from build123d import *

# Parameters (mm, degrees)
F0_W      = 40.221851
F0_H      = 25.612304
F1_DEPTH  = 25.4
F1_FACE_W = 40.22185
F1_FACE_H = 25.612304
F2_DEPTH  = 25.4
F3_R      = 3.681994
F4_DEPTH  = 25.4


with BuildPart() as f1:
    # F0 (on Top) → F1 (new body)
    with BuildSketch(Plane.XY):
        with Locations((4.765831, -2.674487)):
            Rectangle(F0_W, F0_H)
    extrude(amount=F1_DEPTH)

    # F1_face (on face) → F2 (join)
    with BuildSketch(Plane(origin=(4.765831, -2.674487, 25.4), x_dir=(1, 0, 0), z_dir=(0, 0, 1))):
        Rectangle(F1_FACE_W, F1_FACE_H)
    extrude(amount=F2_DEPTH)

    # F3 (on face) → F4 (join)
    with BuildSketch(Plane.XZ.offset(15.480639)):
        with Locations((4.6224, 33.59535)):
            Circle(F3_R)
    extrude(amount=F4_DEPTH)


solid = f1.part
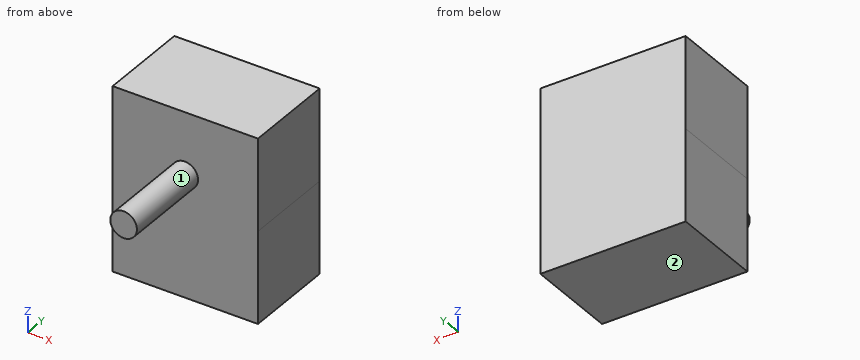
Verification items for the finished model (mm, model axes). Face numbers are marked on the shaded views. A direction names the side the tool comes from. Give positions to 0.01 mm unless a question says otherwise; leave off trailing zeros. Order: outer loops, then holes, each group sorted by start corner. A loop starts at its lowest first (then second) coordinate and runs counter-clockwise, first axis right, second up. Notation, with made-up numbers: M 82,20 L 113,20 A21 ccw 113,29 Z; hole C -20.5,80 d10. An arc over 180 degrees is marked long. Answer as a JSON object with one key per item and string values. Group by question number.
1) Cross-section at A-A (x = 9.5). Enter the section's corners in (y, z).
2) Cross-section at C-C (y = -30). Enter the section's corners in (x, z).
3) Cross-section at D-D (x = 5). Enter the section's corners in (y, z), then the cut area to 3 significant figures.
4) Depth check by flat-ended pin: pin 1 Ø4 at (x, z) = (0, 43.5) entering from -Y; pin 2 Ø4 at (x, y) = (-10.5, -7) entering from -Z; pin 3 Ø1 at (x, y) = (2.5, -35.5) entering from +Z. Enter the tip coordinate at first touch or a pass-through.
5) Scan lines: line 1 along Y through (x, z) = (7.5, 19); line 2 along Z through (x, y) = (5, -31.5); line 3 along Z through (x, y) = (2.5, -36). Record each from-to range of solid material in increasing order. Write a range as [from, to].
6) Cross-section at B-B (z = 46). Enter the section's corners in (x, y).
7) Access from +Z, -Z, +X, -X, +Y, -Y to the whole of each face (thin tool, end or side, straight path). Record for the marked faces 1 and 2.
Result sheet:
{
 "1": {"outline": "M -15.48,0 L 10.13,0 L 10.13,50.8 L -15.48,50.8 Z"},
 "2": {"outline": "C 4.62,33.6 d7.36"},
 "3": {"outline": "M -40.88,29.93 L -15.48,29.93 L -15.48,0 L 10.13,0 L 10.13,50.8 L -15.48,50.8 L -15.48,37.26 L -40.88,37.26 Z", "area": "1,490 mm2"},
 "4": {"pin 1": "stops at y = -15.48", "pin 2": "stops at z = 0", "pin 3": "stops at z = 36.9"},
 "5": {"line 1": "y = [-15.48, 10.13]", "line 2": "z = [29.93, 37.26]", "line 3": "z = [30.59, 36.6]"},
 "6": {"outline": "M -15.35,-15.48 L 24.88,-15.48 L 24.88,10.13 L -15.35,10.13 Z"},
 "7": {"face 1": "-Y", "face 2": "-Z, +X, -X, +Y, -Y"}
}
